Geometry check sheet. Reference: the model listing, model coordinates, mm. Face numbers are marked on the shaded views. Give positions to 0.01 mm unless a question says otherwise; leave off trailing zeros. Write each loop counter-clockwise with the first axis right and the second up, starting at its lowest first coordinate (ties: lowest second). Pieces come first, ordered by that corner, then holes. Notation, with made-up numbers: (89, -3.5) - (119, -3.5) arc R18 ccw to (119, 21.5) - close; hole circle Ø8 at (76, 42.5). An arc over 180 degrees is marked (long way). Use a Markdown table: item, result.
```python
from build123d import *

# Parameters (mm, degrees)
SKETCH2_R               = 6
CUT_EXTRUDE1_DEPTH      = 41
CUT_EXTRUDE1_DEPTH_BACK = 41
SKETCH3_R               = 11
CUT_EXTRUDE2_DEPTH      = 41.0000001
CUT_EXTRUDE2_DEPTH_BACK = 41.0000001


with BuildPart() as part:
    # Sketch1 → Revolve1 (revolve)
    with BuildSketch(Plane.XY):
        Polygon((2, 40), (60, 40), (60, 25), (2, 25), (0, 27), (0, 38), align=None)
    revolve(axis=Axis((0, 0, 0), (1, 0, 0)))

    # Sketch2 → Cut-Extrude1 (cut, two sides)
    with BuildSketch(Plane(origin=(0, 0, 0), x_dir=(1, 0, 0), z_dir=(0, 1, 0))) as cut_extrude1_sk:
        with Locations((20, 0)):
            Circle(SKETCH2_R)
    extrude(amount=CUT_EXTRUDE1_DEPTH, mode=Mode.SUBTRACT)
    extrude(cut_extrude1_sk.sketch, amount=-CUT_EXTRUDE1_DEPTH_BACK, mode=Mode.SUBTRACT)

    # Sketch3 → Cut-Extrude2 (cut, two sides)
    with BuildSketch(Plane.XY) as cut_extrude2_sk:
        with Locations((35, 0)):
            Circle(SKETCH3_R)
    extrude(amount=CUT_EXTRUDE2_DEPTH, mode=Mode.SUBTRACT)
    extrude(cut_extrude2_sk.sketch, amount=-CUT_EXTRUDE2_DEPTH_BACK, mode=Mode.SUBTRACT)


solid = part.part
```
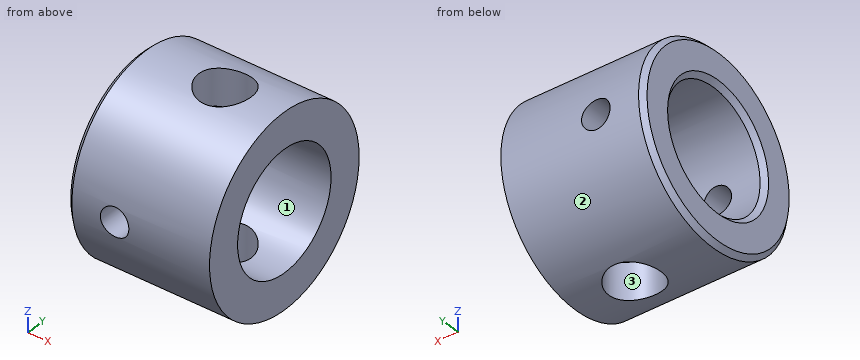
1) Depth check by flat-ended pin: P1, Ø6, axis at y = 27, z = -21.5, coming from the -X side; P2, Ø6, axis at y = 22.5, z = -6, coming from the -X side; P3, Ø1, axis at x = 23, z = -6.5, coming from the -Y side; P4, Ø2, axis at x = 16, z = 13, coming from the +Y side. Enter the tip coordinate at first touch or a pass-through.
Working result:
| item | result |
|---|---|
| P1 | stops at x = 0 |
| P2 | stops at x = 0.71 |
| P3 | stops at y = -39.55 |
| P4 | stops at y = 38.16 |
2) Section check B-B on y = 0. Record the boundary of the cut face in (x, z), then the cut area to 3 significant figures.
Working result:
| item | result |
|---|---|
| outline | (0, -38) - (2, -40) - (24, -40) - (24, -25) - (2, -25) - (0, -27) - close; (0, 27) - (2, 25) - (24, 25) - (24, 40) - (2, 40) - (0, 38) - close; (46, -40) - (60, -40) - (60, -25) - (46, -25) - close; (46, 25) - (60, 25) - (60, 40) - (46, 40) - close |
| area | 1,130 mm² |
3) Section check C-C on x = 35. Record the boundary of the cut face in (y, z), then the cut area to 3 significant figures.
Working result:
| item | result |
|---|---|
| outline | (-11, -38.46) - (-11, -22.45) arc R25 cw to (-11, 22.45) - (-11, 38.46) arc R40 ccw to start; (11, -38.46) arc R40 ccw to (11, 38.46) - (11, 22.45) arc R25 cw to (11, -22.45) - close |
| area | 2,390 mm² |
4) Section check D-D on x = 8. Record the boundary of the cut face in (y, z).
Working result:
| item | result |
|---|---|
| outline | circle Ø80 at (0, 0); hole circle Ø50 at (0, 0) |
5) Mould release check, pull along Z, two halves, no side actions. Record for the marked faces 1, 2 and 3: pulls with the +Z half, pulls with the -Z half, needs draft (parallel to the pull), parting line crosses it, or undercut.
Working result:
| item | result |
|---|---|
| face 1 | undercut |
| face 2 | parting line crosses it |
| face 3 | needs draft |
6) Section check A-A on z = 0. Record the boundary of the cut face in (x, y).
Working result:
| item | result |
|---|---|
| outline | (0, -38) - (2, -40) - (14, -40) - (14, -25) - (2, -25) - (0, -27) - close; (0, 27) - (2, 25) - (14, 25) - (14, 40) - (2, 40) - (0, 38) - close; (26, -40) - (60, -40) - (60, -25) - (26, -25) - close; (26, 25) - (60, 25) - (60, 40) - (26, 40) - close |
7) Material ranges on L1, parallel to X at y = 0, z = 35.75; L2, parallel to Z at x = 28.5, y = 11; L3, parallel to Z at x = 18, y = 0, recorded low to high. Write a range as from..to.
Working result:
| item | result |
|---|---|
| L1 | x = 0..24, 46..60 |
| L2 | z = -38.46..-22.45, 22.45..38.46 |
| L3 | z = -40..-25, 25..40 |
